The figure shows three views and two pictorial views of one solid part (mm, origin at its lowest corner). Answer the questions. A direction names the side the tool comes from. Give positions to 0.01 mm unless a question says otherwise; leave off trailing zeros. Order: outer loops, then holes, each group sorted by start corner. A loop starts at its lowest first (then second) coordinate and runs counter-clockwise, first axis right, second up. Notation, with made-up numbers: (39.5, -36.75) - (55.5, -36.75) arc R8 cw to (55.5, -26.75) - close; hole circle Ø8 at (-21, 75). An arc over 180 degrees is marked (long way). Use a Markdown table: item, result. Add a question column.
1. Which of the six approach directions +Z, -Z, +X, -X, +Y, -Y give full straight-line access (tool end or side, diameter ignored) to the marked faces 4, 5, 6 and 7?
2. For a pull along X with two mould halves and no side action, classify the marked faces 1, 2 and 3 as released by +X, released by -X, zero draft, split by the parting line, or undercut.
3. A cutting plane is placed at B-B on x = 52.5. Determine the outline of the cut face in (y, z).
4. A cutting plane is placed at D-D on x = 26.5. Determine the outline of the cut face in (y, z).
5. Flat-ended cylindrical pins translate along their axes: P1, Ø4.5, axis at x = 30.5, y = 35.5, coming from the -Z side; P2, Ø1.2, axis at x = 29.5, y = 45, coming from the +Z side; P3, Ø0.6, axis at y = 28.5, z = 36, coming from the -X side; P4, Ø10, axis at x = 35.5, y = 21.5, coming from the +Z side. Find the tip coordinate at first contact, or state that the pin passes through.
6. A cutting plane is placed at A-A on z = 42.5. Determine the outline of the cut face in (x, y), and give its area (4 significant figures).
7. A cutting plane is placed at C-C on y = 8. Determine the outline of the cut face in (x, z).
8. Consider L1, parallel to Z at x = 55, y = 27; L2, parallel to X at y = 23.5, z = 16; L3, parallel to Z at x = 30.5, y = 7. Determine where each line is inside the solid, lowest interval first.
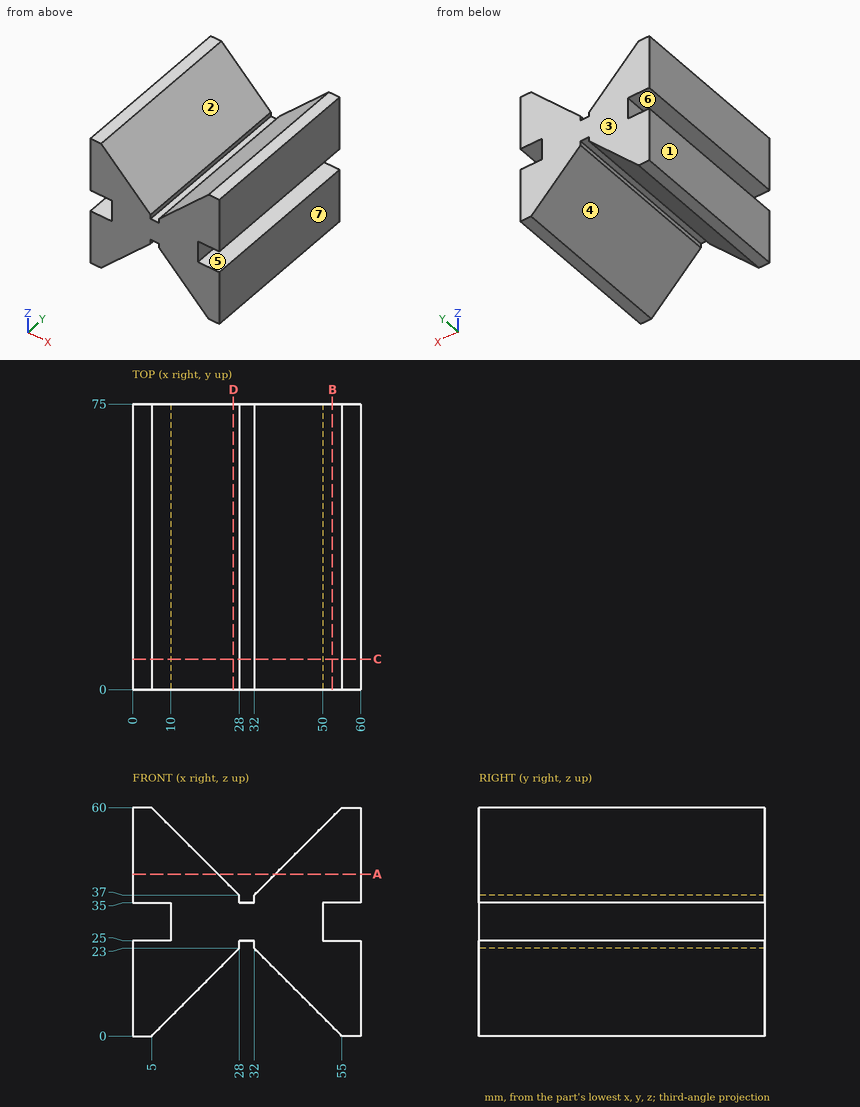
Output values:
| question | item | result |
|---|---|---|
| 1 | face 4 | -Z, +Y, -Y |
| 1 | face 5 | +X, +Y, -Y |
| 1 | face 6 | -X, +Y, -Y |
| 1 | face 7 | +Z, -Z, +X, +Y, -Y |
| 2 | face 1 | released by -X |
| 2 | face 2 | undercut |
| 2 | face 3 | zero draft |
| 3 | outline | (0, 2.5) - (75, 2.5) - (75, 25) - (0, 25) - close; (0, 35) - (75, 35) - (75, 57.5) - (0, 57.5) - close |
| 4 | outline | (0, 21.5) - (75, 21.5) - (75, 38.5) - (0, 38.5) - close |
| 5 | P1 | z = 22.25 |
| 5 | P2 | z = 35 |
| 5 | P3 | x = 0 |
| 5 | P4 | z = 45.5 |
| 6 | outline | (0, 0) - (22.5, 0) - (22.5, 75) - (0, 75) - close; (37.5, 0) - (60, 0) - (60, 75) - (37.5, 75) - close |
| 6 | area | 3,375 mm² |
| 7 | outline | (0, 0) - (5, 0) - (28, 23) - (28, 25) - (32, 25) - (32, 23) - (55, 0) - (60, 0) - (60, 25) - (50, 25) - (50, 35) - (60, 35) - (60, 60) - (55, 60) - (32, 37) - (32, 35) - (28, 35) - (28, 37) - (5, 60) - (0, 60) - (0, 35) - (10, 35) - (10, 25) - (0, 25) - close |
| 8 | L1 | 0 to 25, 35 to 60 |
| 8 | L2 | 0 to 21, 39 to 60 |
| 8 | L3 | 25 to 35 |
